```python
from build123d import *

# Parameters (mm, degrees)
SKETCH3_R          = 3.9
CUT_EXTRUDE1_DEPTH = 10
CIRPATTERN1_COUNT  = 4


with BuildPart() as part:
    # Sketch1 → Revolve1 (revolve)
    with BuildSketch(Plane.XY):
        Polygon((0, 31), (0, 36), (3, 36), (3, 49), (8, 49), (8, 25), (2, 25), (2, 31), align=None)
    revolve(axis=Axis((0, 0, 0), (-1, 0, 0)))

    # Sketch3 → Cut-Extrude1 (cut)
    with BuildSketch(Plane.ZY.offset(-3)):
        with Locations((42.5, 0)):
            Circle(SKETCH3_R)
    cut_extrude1 = extrude(amount=-CUT_EXTRUDE1_DEPTH, mode=Mode.SUBTRACT)

    # CirPattern1: Cut-Extrude1 ×4 about axis
    cirpattern1_axis = Axis((0, 0, 0), (1, 0, 0))
    for i in range(1, CIRPATTERN1_COUNT):
        add(cut_extrude1.rotate(cirpattern1_axis, i * 360 / CIRPATTERN1_COUNT), mode=Mode.SUBTRACT)


solid = part.part
```
CAD build for the part. Positions are in the model's coordinates, mm. A direction names the side the tool comes from. Give positions to 0.01 mm unless a question says otherwise; leave off trailing zeros. Order: outer loops, then holes, each group sorted by start corner. A loop starts at its lowest first (then second) coordinate and runs counter-clockwise, first axis right, second up.
(1) Flat gauge pins, fed straight in: pin 1 (2 mm diameter, centred on x = 3, y = -0.5, fed in from +Z); pin 2 (3 mm diameter, centred on x = 4, z = 6, fed in from +Y); pin 3 (4 mm diameter, centred on y = -22.5, z = 10.5, fed in from +X); pin 4 (1 mm diameter, centred on x = 4.5, y = -28.5, fed in from -Z). Where does each tip first touch, or does it go through?
(2) Drill centre lines: L1, parallel to Y at x = 3.75, z = 1.5; L2, parallel to X at y = -9.5, z = 28.5; L3, parallel to Y at x = 0.85, z = 0. Where is each one in solid material? Low to high.
(3) Mould opens along Y. For faces 1 (the cylindrical face through (5.465, -0.171, -38.604)), 2 (the cylindrical face through (5.54, 26.34, -41.32)), 3 (the flat face through (0, -16, -27)) say: released by +Y, released by -Y, zero draft, split by the parting line, or undercut.
(4) Saw through at A-A, the plane z = 0. Give the cut face in (x, y), then the cut area to 3 significant figures.
(5) Tool access for faces 4 (the cylindrical face through (0.986, -4.036, -30.736)), 5 (the cylindrical face through (5.465, 38.604, -0.171)): list every direction of +Z, -Z, +X, -X, +Y, -Y with a clear straight run to the whole face (end or side of a thin tool).
(6) Saw through at C-C, the plane y = -42.5. Give the cut face in (x, z).
Results found:
1. pin 1: stops at z = 49
1. pin 2: stops at y = 48.79
1. pin 3: stops at x = 8
1. pin 4: stops at z = -40.21
2. L1: y = -48.98 to -46.1, -38.9 to -24.95, 24.95 to 38.9, 46.1 to 48.98
2. L2: x = 2 to 8
2. L3: y = -36 to -31, 31 to 36
3. face 1: undercut
3. face 2: split by the parting line
3. face 3: zero draft
4. outline: (0, -36) - (3, -36) - (3, -38.6) - (8, -38.6) - (8, -25) - (2, -25) - (2, -31) - (0, -31) - close; (0, 31) - (2, 31) - (2, 25) - (8, 25) - (8, 38.6) - (3, 38.6) - (3, 36) - (0, 36) - close; (3, -49) - (8, -49) - (8, -46.4) - (3, -46.4) - close; (3, 46.4) - (8, 46.4) - (8, 49) - (3, 49) - close
4. area: 204 mm2
5. face 4: -X
5. face 5: +X, -X
6. outline: (3, -24.39) - (8, -24.39) - (8, -3.9) - (3, -3.9) - close; (3, 3.9) - (8, 3.9) - (8, 24.39) - (3, 24.39) - close
